Source: CAD feature listing. Evaluate the final solid. Frame: model axes, mm. A direction names the side the tool comes from. Coordinates: 2 decimals unless noted, no trailing zeros. Write each loop counter-clockwise with the first axis right and the second up, starting at its lowest first coordinate (ties: lowest second). Pieces come first, ordered by that corner, then holes. Notation, with made-up numbers: (-23.75, 59.5) - (10.25, 59.5) arc R17 cw to (10.25, 69.5) - close; hole circle Ø4 at (7.5, -11.75). An arc over 180 degrees is marked (long way). One line per item, written item: value.
from build123d import *

# Parameters (mm, degrees)
BOSS_EXTRUDE1_DEPTH = 50.8
CUT_EXTRUDE1_DEPTH  = 2.27


with BuildPart() as part:
    # Sketch2 → Boss-Extrude1 (new body, symmetric)
    with BuildSketch(Plane(origin=(0, 0, 0), x_dir=(1, 0, 0), z_dir=(0, 1, 0))):
        with BuildLine():
            Line((-5.334, 0), (20.066, 0))
            ThreePointArc((20.066, 0), (20.335407684, -0.111592316), (20.447, -0.381))
            Line((20.447, -0.381), (20.447, -0.889))
            ThreePointArc((20.447, -0.889), (20.335407684, -1.158407684), (20.066, -1.27))
            Line((20.066, -1.27), (1.651, -1.27))
            ThreePointArc((1.651, -1.27), (1.381592316, -1.381592316), (1.27, -1.651))
            Line((1.27, -1.651), (1.27, -5.461))
            ThreePointArc((1.27, -5.461), (1.158407684, -5.730407684), (0.889, -5.842))
            Line((0.889, -5.842), (-0.76996875, -5.842))
            ThreePointArc((-0.76996875, -5.842), (-0.904672592, -5.866607134), (-1.021976563, -5.93725))
            ThreePointArc((-1.021976563, -5.93725), (-2.921, -5.08), (-1.021976563, -4.22275))
            ThreePointArc((-1.021976563, -4.22275), (-0.904672592, -4.293392866), (-0.76996875, -4.318))
            Line((-0.76996875, -4.318), (-0.381, -4.318))
            ThreePointArc((-0.381, -4.318), (-0.111592316, -4.206407684), (0, -3.937))
            Line((0, -3.937), (0, -1.651))
            ThreePointArc((0, -1.651), (-0.111592316, -1.381592316), (-0.381, -1.27))
            Line((-0.381, -1.27), (-5.334, -1.27))
            ThreePointArc((-5.334, -1.27), (-5.603407684, -1.158407684), (-5.715, -0.889))
            Line((-5.715, -0.889), (-5.715, -0.381))
            ThreePointArc((-5.715, -0.381), (-5.603407684, -0.111592316), (-5.334, 0))
        make_face()
    extrude(amount=BOSS_EXTRUDE1_DEPTH, both=True)

    # Sketch3 → Cut-Extrude1 (cut, through all)
    with BuildSketch(Plane.XY.offset(1.27)):
        with BuildLine():
            Line((11.71575, 2.38125), (13.30325, 2.38125))
            ThreePointArc((13.30325, 2.38125), (15.6845, 0), (13.30325, -2.38125))
            Line((13.30325, -2.38125), (11.71575, -2.38125))
            ThreePointArc((11.71575, -2.38125), (9.3345, 0), (11.71575, 2.38125))
        make_face()
    extrude(amount=-CUT_EXTRUDE1_DEPTH, mode=Mode.SUBTRACT)


solid = part.part
1) Reachability of faces 4 (the flat face through (1.27, 1, 4)), 5 (the cylindrical face through (9.335, -0.052, 0.644)), 6 (the flat face through (-3, 1, 1.27)) from +Z, -Z, +X, -X, +Y, -Y: full face, straight path, thin tool, end or side. Return the list, or none.
Values found:
face 4: +Z, +X, +Y, -Y
face 5: +Z, -Z
face 6: -X, +Y, -Y
2) Contact query for flat-ended pins moving along their axis: P1, Ø1, axis at x = 17, y = 36.5, coming from the +Z side; P2, Ø1.3, axis at x = 0.5, y = 2.5, coming from the +Z side; P3, Ø1.5, axis at x = -3.5, y = 20, coming from the +Z side; P4, Ø10, axis at x = 0.5, y = 31, coming from the +Z side. Output: stop coordinate, or through.
Values found:
P1: z = 1.27
P2: z = 5.84
P3: z = 5.68
P4: z = 6.22
3) Section query C-C on x = 7.5. Output: boundary loops of the cut face in (y, z), then the cut area to 3 significant figures.
Values found:
outline: (-50.8, 0) - (50.8, 0) - (50.8, 1.27) - (-50.8, 1.27) - close
area: 129 mm2
4) Draft query along Y for faces 1 (the cylindrical face through (15.684, 0.052, 0.644)), 2 (the flat face through (5, 50.8, 1)), 3 (the flat face through (5, -50.8, 1)). Return one class per face: released by +Y, released by -Y, zero draft, split by the parting line, or undercut.
Values found:
face 1: undercut
face 2: released by +Y
face 3: released by -Y
5) Section query B-B on y = 12.5. Output: boundary loops of the cut face in (x, z) (3 decimals), then the cut area to 3 significant figures.
Values found:
outline: (-5.715, 0.381) arc R0.381 ccw to (-5.334, 0) - (20.066, 0) arc R0.381 ccw to (20.447, 0.381) - (20.447, 0.889) arc R0.381 ccw to (20.066, 1.27) - (1.651, 1.27) arc R0.381 cw to (1.27, 1.651) - (1.27, 5.461) arc R0.381 ccw to (0.889, 5.842) - (-0.77, 5.842) arc R0.381 cw to (-1.022, 5.937) arc R1.143 ccw (long way) to (-1.022, 4.223) arc R0.381 cw to (-0.77, 4.318) - (-0.381, 4.318) arc R0.381 cw to (0, 3.937) - (0, 1.651) arc R0.381 cw to (-0.381, 1.27) - (-5.334, 1.27) arc R0.381 ccw to (-5.715, 0.889) - close
area: 44.2 mm2
6) Material intervals for line 1 (Z direction, x = -1, y = -42); line 2 (Z direction, x = 2.75, y = 26), sorted ascending.
Values found:
line 1: 0 to 1.27, 4.24 to 5.92
line 2: 0 to 1.27
